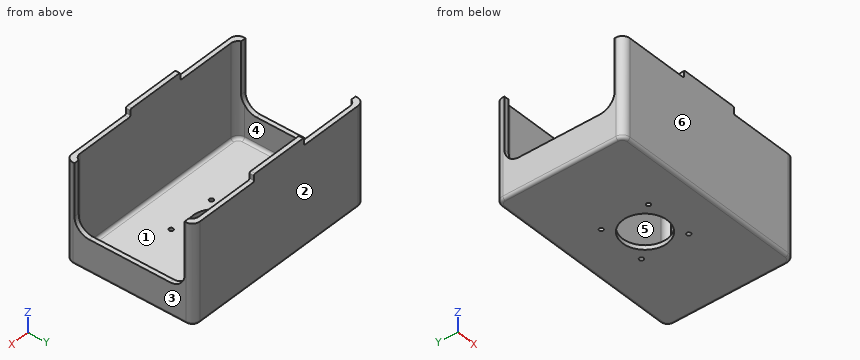
from build123d import *

# Parameters (mm, degrees)
F0_R     = 3
F0_R_2   = 1.4
F0_R_3   = 15
F0_R_4   = 1.5
F1_DEPTH = 3
F0_W     = 65
F0_H     = 3
F2_DEPTH = 67
F4_DEPTH = 136.001
F5_W     = 39.8
F5_H     = 3
F6_W     = 39.8
F6_H     = 3
F7_DEPTH = 5
F8_R     = 1
F9_R     = 5
F10_R    = 2


# Not quite as in the source:
# - a feature names something its author has since deleted; it is built from what else it names


with BuildPart() as f1:
    # F0 (on Top) → F1 (new body)
    with BuildSketch(Plane.XY):
        Polygon((-60.3749420391, 27.6098903269), (-60.3749420391, 7), (-15.3749420391, 7), (-15.3749420391, 12), (24.6250579609, 12), (24.6250579609, 7), (69.6250579609, 7), (69.6250579609, 53.4099719524), (69.6250579609, 87.5), (4.6250579609, 87.5), (-60.3749420391, 87.5), (-60.3749420391, 71.25), align=None)
        with Locations((-30.3749420391, 23.25)):
            Circle(F0_R, mode=Mode.SUBTRACT)
        with Locations((-11.3749420391, 31.25)):
            Circle(F0_R_2, mode=Mode.SUBTRACT)
        with Locations((20.6250579609, 31.25)):
            Circle(F0_R_2, mode=Mode.SUBTRACT)
        with Locations((52.6250579609, 23.25)):
            Circle(F0_R, mode=Mode.SUBTRACT)
        with Locations((-11.3749420391, 63.25)):
            Circle(F0_R_2, mode=Mode.SUBTRACT)
        with BuildLine():
            ThreePointArc((-27.3749420391, 71.25), (-30.3749420391, 68.25), (-33.3749420391, 71.25))
            ThreePointArc((-33.3749420391, 71.25), (-30.3749420391, 74.25), (-27.3749420391, 71.25))
        make_face(mode=Mode.SUBTRACT)
        with Locations((4.6250579609, 47.25)):
            Circle(F0_R_3, mode=Mode.SUBTRACT)
        with Locations((20.6250579609, 63.25)):
            Circle(F0_R_2, mode=Mode.SUBTRACT)
        with Locations((52.6250579609, 71.25)):
            Circle(F0_R, mode=Mode.SUBTRACT)
        Polygon((-15.3749420391, 12), (-15.3749420391, 7), (14.8769766092, 7), (24.6250579609, 7), (24.6250579609, 12), align=None)
        with BuildLine():
            ThreePointArc((-27.3749420391, 71.25), (-30.3749420391, 74.25), (-33.3749420391, 71.25))
            ThreePointArc((-33.3749420391, 71.25), (-30.3749420391, 68.25), (-27.3749420391, 71.25))
        make_face()
        with BuildLine():
            ThreePointArc((-28.8749420391, 71.25), (-30.3749420391, 69.75), (-31.8749420391, 71.25))
            ThreePointArc((-31.8749420391, 71.25), (-30.3749420391, 72.75), (-28.8749420391, 71.25))
        make_face(mode=Mode.SUBTRACT)
        with BuildLine():
            ThreePointArc((-28.8749420391, 71.25), (-30.3749420391, 72.75), (-31.8749420391, 71.25))
            ThreePointArc((-31.8749420391, 71.25), (-30.3749420391, 69.75), (-28.8749420391, 71.25))
        make_face()
        with Locations((52.6250579609, 71.25)):
            Circle(F0_R)
        with Locations((52.6250579609, 71.25)):
            Circle(F0_R_4, mode=Mode.SUBTRACT)
        with Locations((52.6250579609, 71.25)):
            Circle(F0_R_4)
        with Locations((52.6250579609, 23.25)):
            Circle(F0_R)
        with Locations((52.6250579609, 23.25)):
            Circle(F0_R_4, mode=Mode.SUBTRACT)
        with Locations((52.6250579609, 23.25)):
            Circle(F0_R_4)
        with Locations((-30.3749420391, 23.25)):
            Circle(F0_R)
        with Locations((-30.3749420391, 23.25)):
            Circle(F0_R_4, mode=Mode.SUBTRACT)
        with Locations((-30.3749420391, 23.25)):
            Circle(F0_R_4)
    extrude(amount=F1_DEPTH)

    # F0 (on Top) → F2 (join)
    with BuildSketch(Plane.XY):
        Polygon((-63.3749420391, 27.6098903269), (-60.3749420391, 27.6098903269), (-60.3749420391, 71.25), (-60.3749420391, 87.5), (-60.3749420391, 90.5), (-63.3749420391, 90.5), align=None)
        with Locations((-27.8749420391, 89)):
            Rectangle(F0_W, F0_H)
        with Locations((37.1250579609, 89)):
            Rectangle(F0_W, F0_H)
        Polygon((69.6250579609, 87.5), (69.6250579609, 53.4099719524), (72.6250579609, 53.4099719524), (72.6250579609, 90.5), (69.6250579609, 90.5), align=None)
        Polygon((69.6250579609, 7), (69.6250579609, 4), (72.6250579609, 4), (72.6250579609, 53.4099719524), (69.6250579609, 53.4099719524), align=None)
        Polygon((14.8769766092, 4), (69.6250579609, 4), (69.6250579609, 7), (24.6250579609, 7), (14.8769766092, 7), align=None)
        Polygon((-60.3749420391, 7), (-60.3749420391, 4), (14.8769766092, 4), (14.8769766092, 7), (-15.3749420391, 7), align=None)
        Polygon((-63.3749420391, 4), (-60.3749420391, 4), (-60.3749420391, 7), (-60.3749420391, 27.6098903269), (-63.3749420391, 27.6098903269), align=None)
    extrude(amount=F2_DEPTH)

    # F3 (on face) → F4 (cut, through all)
    with BuildSketch(Plane(origin=(-63.3749420391, 0, 0), x_dir=(0, -1, 0), z_dir=(-1, 0, 0))):
        with BuildLine():
            ThreePointArc((-20, 21.9706685841), (-12.9289321881, 24.8996007722), (-10, 31.9706685841))
            ThreePointArc((-10, 31.9706685841), (-20, 41.9706685841), (-30, 31.9706685841))
            ThreePointArc((-30, 31.9706685841), (-27.0710678119, 24.8996007722), (-20, 21.9706685841))
        make_face()
        with BuildLine():
            ThreePointArc((-30, 31.9706685841), (-20, 41.9706685841), (-10, 31.9706685841))
            Line((-10, 31.9706685841), (-10, 67))
            Line((-10, 67), (-30, 67))
            Line((-30, 67), (-30, 31.9706685841))
        make_face()
        with BuildLine():
            ThreePointArc((-74.5, 21.9706685841), (-67.4289321881, 24.8996007722), (-64.5, 31.9706685841))
            ThreePointArc((-64.5, 31.9706685841), (-74.5, 41.9706685841), (-84.5, 31.9706685841))
            ThreePointArc((-84.5, 31.9706685841), (-81.5710678119, 24.8996007722), (-74.5, 21.9706685841))
        make_face()
        with BuildLine():
            Line((-64.5, 31.9706685841), (-30, 31.9706685841))
            Line((-30, 31.9706685841), (-30, 67))
            Line((-30, 67), (-84.5, 67))
            Line((-84.5, 67), (-84.5, 31.9706685841))
            ThreePointArc((-84.5, 31.9706685841), (-74.5, 41.9706685841), (-64.5, 31.9706685841))
        make_face()
        with BuildLine():
            ThreePointArc((-20, 21.9706685841), (-27.0710678119, 24.8996007722), (-30, 31.9706685841))
            Line((-30, 31.9706685841), (-64.5, 31.9706685841))
            ThreePointArc((-64.5, 31.9706685841), (-67.4289321881, 24.8996007722), (-74.5, 21.9706685841))
            Line((-74.5, 21.9706685841), (-20, 21.9706685841))
        make_face()
    extrude(amount=-F4_DEPTH, mode=Mode.SUBTRACT)

    # F5 (on face) + F6 (on face) → F7 (join)
    with BuildSketch(Plane.XY.offset(67)):
        with Locations((4.6250579609, 5.5)):
            Rectangle(F5_W, F5_H)
    with BuildSketch(Plane.XY.offset(67)):
        with Locations((4.6250579609, 89)):
            Rectangle(F6_W, F6_H)
    extrude(amount=F7_DEPTH)

    # F8
    f8_edges = [f1.edges().sort_by_distance(p)[0] for p in [
        (-15.274942, 5.5, 67),
        (-15.274942, 5.5, 72),
        (24.525058, 5.5, 72),
        (24.525058, 5.5, 67),
        (-15.274942, 89, 67),
        (-15.274942, 89, 72),
        (24.525058, 89, 72),
        (24.525058, 89, 67),
    ]]
    fillet(f8_edges, radius=F8_R)

    # F9
    f9_edges = [f1.edges().sort_by_distance(p)[0] for p in [
        (72.625058, 4, 33.5),
        (72.625058, 90.5, 33.5),
        (-63.374942, 90.5, 33.5),
        (-63.374942, 4, 33.5),
        (-60.374942, 7, 35),
        (-60.374942, 87.5, 35),
        (69.625058, 87.5, 35),
        (69.625058, 7, 35),
    ]]
    fillet(f9_edges, radius=F9_R)

    # F10
    f10_edges = [f1.edges().sort_by_distance(p)[0] for p in [
        (4.625058, 87.5, 3),
        (4.625058, 4, 0),
    ]]
    fillet(f10_edges, radius=F10_R)


solid = f1.part
Could you check a few things on this model? Use its own coordinates, in mm. Face numbers are marked on the shaded views. A direction names the side the tool comes from. Round coordinates to 2 decimals unless told otherwise and drop trailing zeros. Write each loop counter-clockwise with the first axis right and the second up, starting at its lowest first coordinate (ties: lowest second). Pieces come first, ordered by that corner, then holes. Notation, with made-up numbers: (61, 8) - (79, 8) arc R12 cw to (79, 20) - close; hole circle Ø2 at (18.5, 52). An arc over 180 degrees is marked (long way). Put each result on its own line as item: value. Start each with the question number.
(1) Will these pins go through, and if not, where does the flat tip stop? pin 1 (0.9 mm diameter, centred on x = 71, y = 50, fed in from +Z); pin 2 (1.7 mm diameter, centred on x = 70, z = 46, fed in from +Y); pin 3 (2 mm diameter, centred on x = -11.37, y = 63.25, fed in from +Z); pin 4 (0.9 mm diameter, centred on y = 89, z = 69.5, fed in from -X).
(2) I want a section at C-C, the plane z = 46. Please give me the cut outline in (x, y).
(3) I want a section at D-D, the plane x = -28.5. Please give me the cut outline in (y, z).
(4) Thinking about a two-plate mould opening in Y: for the marked faces 1, 2, 3 and 4, which applies, released by +Y, released by -Y, zero draft, split by the parting line, or undercut?
(5) For the marked faces 5 and 6, which set-ups out of +Z, -Z, +X, -X, +Y, -Y let a thin tool reach every point of the face, with its end or its side?
(6) I want a section at A-A, the plane y = 47.25. Please give me the cut outline in (x, z), plus the area to 3 significant figures.
(7) I need wall thicknesses on probe 1 along X at (y, z) = (63, 2); probe 2 along Y at (x, z) = (47, 60); probe 3 along X at (y, z) = (65, 19). Which ranges of each line are inside material? Lowest first, please.
(8) I want a section at B-B, the plane z = 9. Please give me the cut outline in (x, y).
Here are the results:
1. pin 1: stops at z = 21.97
1. pin 2: stops at y = 90.26
1. pin 3: passes through
1. pin 4: stops at x = -15.27
2. outline: (-63.37, 9) arc R5 ccw to (-58.37, 4) - (67.63, 4) arc R5 ccw to (72.63, 9) - (72.63, 10) - (69.21, 10) arc R5 cw to (64.63, 7) - (-55.37, 7) arc R5 cw to (-59.96, 10) - (-63.37, 10) - close; (-63.37, 84.5) - (-59.96, 84.5) arc R5 cw to (-55.37, 87.5) - (64.63, 87.5) arc R5 cw to (69.21, 84.5) - (72.63, 84.5) - (72.63, 85.5) arc R5 ccw to (67.63, 90.5) - (-58.37, 90.5) arc R5 ccw to (-63.37, 85.5) - close
3. outline: (4, 2) arc R2 ccw to (6, 0) - (88.5, 0) arc R2 ccw to (90.5, 2) - (90.5, 67) - (87.5, 67) - (87.5, 5) arc R2 cw to (85.5, 3) - (9, 3) arc R2 cw to (7, 5) - (7, 67) - (4, 67) - close
4. face 1: undercut
4. face 2: released by +Y
4. face 3: zero draft
4. face 4: undercut
5. face 5: +Z
5. face 6: +Z, -Z, +X, -X, -Y
6. outline: (-63.37, 2) arc R2 ccw to (-61.37, 0) - (-10.37, 0) - (-10.37, 3) - (-58.37, 3) arc R2 cw to (-60.37, 5) - (-60.37, 21.97) - (-63.37, 21.97) - close; (19.63, 0) - (70.63, 0) arc R2 ccw to (72.63, 2) - (72.63, 21.97) - (69.63, 21.97) - (69.63, 5) arc R2 cw to (67.63, 3) - (19.63, 3) - close
6. area: 432 mm^2
7. probe 1: x = -63.37 to -12.75, -10 to 19.25, 22 to 72.63
7. probe 2: y = 4 to 7, 87.5 to 90.5
7. probe 3: x = -63.37 to -60.37, 69.63 to 72.63
8. outline: (-63.37, 9) arc R5 ccw to (-58.37, 4) - (67.63, 4) arc R5 ccw to (72.63, 9) - (72.63, 85.5) arc R5 ccw to (67.63, 90.5) - (-58.37, 90.5) arc R5 ccw to (-63.37, 85.5) - close; hole (-60.37, 12) arc R5 ccw to (-55.37, 7) - (64.63, 7) arc R5 ccw to (69.63, 12) - (69.63, 82.5) arc R5 ccw to (64.63, 87.5) - (-55.37, 87.5) arc R5 ccw to (-60.37, 82.5) - close
